For this review, take the finished solid that the model builds, in its own axes (mm). Give positions to 0.01 mm unless a question says otherwise; leave off trailing zeros. Write each loop counter-clockwise with the first axis right and the second up, starting at its lowest first coordinate (ties: lowest second). Pieces come first, ordered by that corner, then holes.
1) Draft analysis for pull direction X (two halves, no side actions). For faces 1 (the face through (-42.693, 2.465, -1.107)), 2 (the face through (-53, 6, -6)), 3 (the face through (-55.995, 2.553, -0.215)), state which applies: pulls with the +X half, pulls with the -X half, needs draft (parallel to the pull), parting line crosses it, or undercut.
2) Wall thickness on line 1 along X through (y, z) = (3.25, 2.75); line 2 along Z through (x, y) = (-51, 1.5); line 3 along X through (y, z) = (2.1, 0.5): over which ranges is each line inside the solid? List them lowest first.
3) We need section C-C on y = 4. Give the boundary of the cut face in (x, z), and give its area (3 significant figures).
4) We need section B-B on y = 1.4. Give the boundary of the cut face in (x, z), and give its area (3 significant figures).
5) We need section A-A on z = 0. Give the boundary of the cut face in (x, y).
6) For P1, Ø3, axis at x = -58, y = 3.5, coming from the -Z side; P2, Ø1.5, axis at x = -46.5, z = -7, coming from the +Y side, all flat-tipped, find the tip position at first contact; note any pin that passes through.
from build123d import *

# Parameters (mm, degrees)
SKETCH1_R           = 8.5
BOSS_EXTRUDE1_DEPTH = 6
FILLET2_R           = 1
SKETCH2_R           = 5
CUT_EXTRUDE4_DEPTH  = 6
CUT_EXTRUDE4_DRAFT  = -2
FILLET5_R           = 1


with BuildPart() as part:
    # Sketch1 → Boss-Extrude1 (new body)
    with BuildSketch(Plane(origin=(0, 0, 0), x_dir=(1, 0, 0), z_dir=(0, 1, 0))):
        with Locations(Location((-51.120170416, 0, 0), (0, 0, 270))):
            Circle(SKETCH1_R)
    extrude(amount=BOSS_EXTRUDE1_DEPTH)

    # Fillet2
    fillet2_edges = [part.edges().sort_by_distance(p)[0] for p in [
        (-51.120170416, 6, -8.5),
    ]]
    fillet(fillet2_edges, radius=FILLET2_R)


with BuildPart() as cut_extrude4_tool:
    # Sketch2 → Cut-Extrude4 (with draft: the straight prism first)
    with BuildSketch(Plane(origin=(0, 6, 0), x_dir=(1, 0, 0), z_dir=(0, 1, 0))):
        with Locations((-51.120170416, 0)):
            Circle(SKETCH2_R)
    extrude(amount=-CUT_EXTRUDE4_DEPTH)
    # Cut-Extrude4: the draft: its side faces are tilted about the plane it starts from
    cut_extrude4_sides = [cut_extrude4_tool.faces().sort_by_distance(p)[0] for p in [
        (-56.120170416, 3, 0),
    ]]
    draft(cut_extrude4_sides, Plane(origin=(0, 6, 0), x_dir=(1, 0, 0), z_dir=(0, 1, 0)), CUT_EXTRUDE4_DRAFT)


with BuildPart() as part_1:
    add(part.part)

    # Cut-Extrude4: cut by cut_extrude4_tool
    add(cut_extrude4_tool.part, mode=Mode.SUBTRACT)

    # Fillet5
    fillet5_edges = [part_1.edges().sort_by_distance(p)[0] for p in [
        (-56.120170416, 6, 0),
    ]]
    fillet(fillet5_edges, radius=FILLET5_R)


solid = part_1.part
Results list:
1. face 1: parting line crosses it
1. face 2: needs draft
1. face 3: undercut
2. line 1: x = -59.16 to -55.18, -47.06 to -43.08
2. line 2: z = -8.5 to -4.84, 4.84 to 8.5
2. line 3: x = -59.61 to -55.96, -46.28 to -42.63
3. outline: circle Ø17 at (-51.12, 0); hole circle Ø9.86 at (-51.12, 0)
3. area: 151 mm2
4. outline: circle Ø17 at (-51.12, 0); hole circle Ø9.68 at (-51.12, 0)
4. area: 153 mm2
5. outline: (-59.62, 0) - (-55.91, 0) - (-56.09, 5.03) arc R1 ccw to (-57.09, 6) - (-58.62, 6) arc R1 ccw to (-59.62, 5) - close; (-46.33, 0) - (-42.62, 0) - (-42.62, 5) arc R1 ccw to (-43.62, 6) - (-45.15, 6) arc R1 ccw to (-46.15, 5.03) - close
6. P1: stops at z = -6.58
6. P2: stops at y = 5.99
